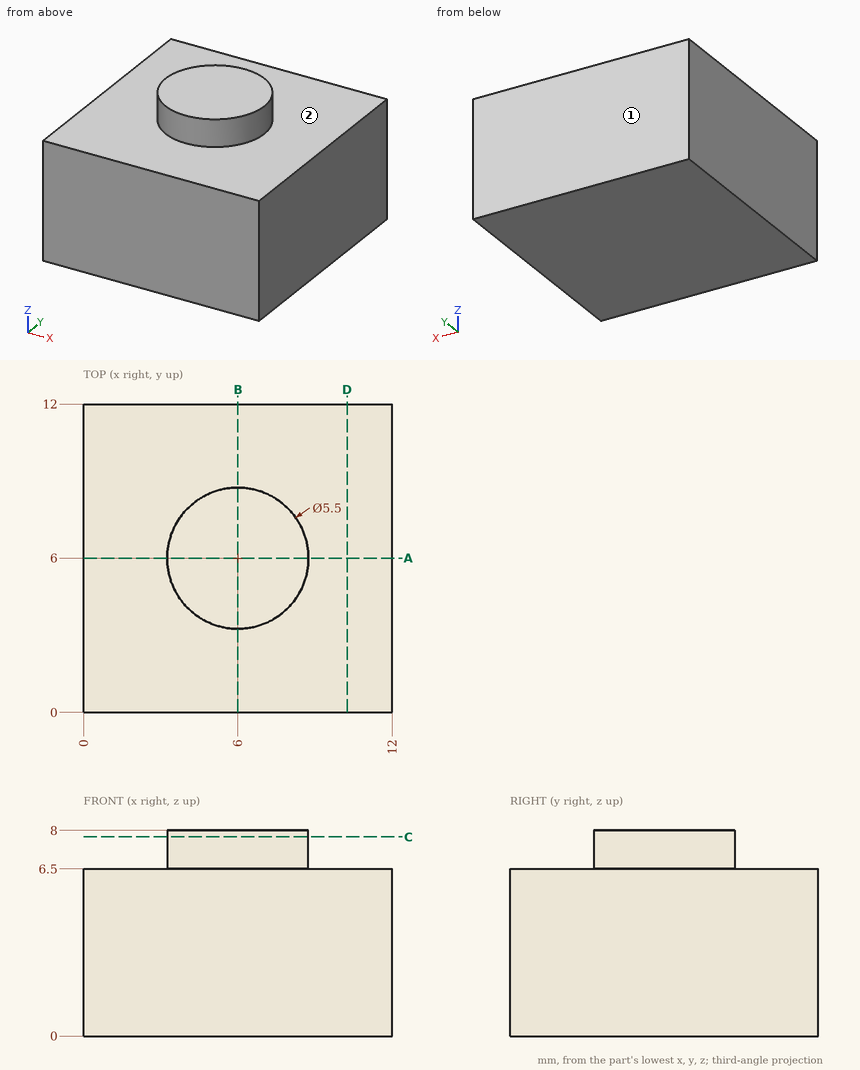
For this review, use the dimensioned drawing (mm, ordinates from the lowest corner) and the shaded views. A direction names the side the tool comes from. Round coordinates to 2 decimals unless told otherwise and drop trailing zeros. Loops run counter-clockwise (first coordinate to the right, second up) from the corner with the lowest first, then second, coordinate; pieces in that order, holes last. Notation, with made-up numbers: (11.5, 15.25) -> (18.5, 15.25) arc R29 cw to (18.5, 41.25) -> close; hole circle Ø5 at (56.5, 46.25). An arc over 180 degrees is marked (long way). Write item = value, one per line. Start each with the question number.
Item 1: Take a section at D-D on x = 10.25. Give the boundary of the cut face in (y, z).
Item 2: Take a section at A-A on y = 6. Give the boundary of the cut face in (x, z).
Item 3: Take a section at C-C on z = 7.75. Give the boundary of the cut face in (x, y).
Item 4: To check wall thickness, follow L1, parallel to Z at x = 5.75, y = 11. State the ranges of the line that lie inside material, in increasing order.
Item 5: For the marked faces 1 and 2, list the 3-axis set-ups (+Z, -Z, +X, -X, +Y, -Y) from which the entire face can be reached by the end or side of a thin tool; tool diameter is ignored.
Result:
q1.outline = (0, 0) -> (12, 0) -> (12, 6.5) -> (0, 6.5) -> close
q2.outline = (0, 0) -> (12, 0) -> (12, 6.5) -> (8.75, 6.5) -> (8.75, 8) -> (3.25, 8) -> (3.25, 6.5) -> (0, 6.5) -> close
q3.outline = circle Ø5.5 at (6, 6)
q4.L1 = 0 to 6.5
q5.face_1 = +Z, -Z, +X, -X, +Y
q5.face_2 = +Z
